The listing builds one solid part. Answer for the finished solid, in the listing's coordinates (mm). A direction names the side the tool comes from. Give positions to 0.01 mm unless a question says otherwise; leave off trailing zeros. Loops run counter-clockwise (first coordinate to the right, second up) from the corner with the lowest first, then second, coordinate; pieces in that order, holes last.
Item 1: The mould has two halves that part along X. Classify faces 1 (the face through (-6.43, 3.77, -7.44)), 2 (the face through (0, 2.8, 0)), 3 (the face through (4, 0, 0)): pulls with the +X half, pulls with the -X half, needs draft (parallel to the pull), parting line crosses it, or undercut.
Item 2: Each of these flat-tipped pins is pushed along its axis until it touches: pin 1 Ø0.5 at (y, z) = (0.5, 2) entering from -X; pin 2 Ø1 at (x, z) = (6, 1) entering from +Y; pin 3 Ø1.4 at (y, z) = (2, 1) entering from +X. Where does it stop, or does it pass through?
Item 3: Section B-B, the plane z = 0.5 is taken. Give the vertices of the cut face in (x, y), and give its area (3 significant figures).
Item 4: A tool of negligible diameter and unlimited length cuts with its end or side. For faces 4 (the face through (-6.43, 3.77, 7.44)), 5 (the face through (1.95, 2, 0)), 6 (the face through (2, 6, -1.5)), 7 (the face through (0, 3, -7.5)), 8 (the face through (2, 6, 1.5)), from which of +Z, -Z, +X, -X, +Y, -Y can it reach the whole face along a straight path? Write none if from no direction.
Item 5: Consider line 1 along Z through (x, y) = (1.25, 6.25); line 2 along Y through (x, z) = (1, -1.75); line 3 along X through (y, z) = (2, -5). Determine where each line is inside the solid, lowest interval first.
Item 6: Section A-A, the plane z = 2.75 is taken. Give the vertices of the cut face in (x, y).
from build123d import *

# Parameters (mm, degrees)
EXTRUDE_1_DEPTH      = 7.5
EXTRUDE_1_DEPTH_BACK = 7.5
EXTRUDE_2_DEPTH      = 1.5
EXTRUDE_2_DEPTH_BACK = 1.5
EXTRUDE_3_DEPTH      = 2
EXTRUDE_3_DEPTH_BACK = 2
CUT_EXTRUDE_1_DEPTH  = 16.207955299
FILLET_1_R           = 0.2
FILLET_2_R           = 0.1


with BuildPart() as part:
    # 草图1 → 凸台-拉伸1 (new, two sides: drawn at the far end of the back side and taken through both)
    with BuildSketch(Plane.XY.offset(-EXTRUDE_1_DEPTH_BACK)):
        with BuildLine():
            Line((-7.5, 0), (-1.5, 0))
            Line((-1.5, 0), (-1.5, 0.677124344))
            ThreePointArc((-1.5, 0.677124344), (-1.780042303, 1.088161527), (-1.95, 1.555590279))
            Line((-1.95, 1.555590279), (-1.95, 2.8))
            Line((-1.95, 2.8), (1.95, 2.8))
            Line((1.95, 2.8), (1.95, 1.555590279))
            ThreePointArc((1.95, 1.555590279), (1.780042303, 1.088161527), (1.5, 0.677124344))
            Line((1.5, 0.677124344), (1.5, 0))
            Line((1.5, 0), (7.5, 0))
            Line((7.5, 0), (8.53527618, 3.863703305))
            Line((8.53527618, 3.863703305), (-5.459914348, 7.613703305))
            Line((-5.459914348, 7.613703305), (-7.5, 0))
        make_face()
    extrude(amount=EXTRUDE_1_DEPTH + EXTRUDE_1_DEPTH_BACK)

    # 草图2 → 凸台-拉伸2 (add, two sides: drawn at the far end of the back side and taken through both)
    with BuildSketch(Plane.XY.offset(-EXTRUDE_2_DEPTH_BACK)):
        Polygon((0.088792177, 6.126931873), (2.986569656, 5.350474738), (3.245388701, 6.316400564), (0.347611222, 7.092857699), align=None)
    extrude(amount=EXTRUDE_2_DEPTH + EXTRUDE_2_DEPTH_BACK)

    # 草图3 → 凸台-拉伸3 (add, two sides: drawn at the far end of the back side and taken through both)
    with BuildSketch(Plane.XY.offset(-EXTRUDE_3_DEPTH_BACK)):
        with BuildLine():
            Line((2.184728529, 8.153517871), (4.06828389, 7.648820733))
            Line((4.06828389, 7.648820733), (3.823852668, 6.736590993))
            ThreePointArc((3.823852668, 6.736590993), (3.538706676, 6.329077778), (3.161822332, 6.004526629))
            Line((3.161822332, 6.004526629), (0.264044853, 6.780983765))
            ThreePointArc((0.264044853, 6.780983765), (0.099929011, 7.250495477), (0.056741946, 7.745985269))
            Line((0.056741946, 7.745985269), (0.301173168, 8.658215009))
            Line((0.301173168, 8.658215009), (2.184728529, 8.153517871))
        make_face()
    extrude(amount=EXTRUDE_3_DEPTH + EXTRUDE_3_DEPTH_BACK)

    # 草图4 → 切除-拉伸1 (cut, through all)
    with BuildSketch(Plane(origin=(-1.883555361, 0.504697138, 0), x_dir=(0, 0, 1), z_dir=(-0.9659258262890692, 0.2588190451025178, 0))):
        with BuildLine():
            Line((1.95, 8.441142838), (2, 8.441142838))
            Line((2, 8.441142838), (2, 6.618267183))
            Line((2, 6.618267183), (1.5, 6.618267183))
            ThreePointArc((1.5, 6.618267183), (1.780042303, 7.029304366), (1.95, 7.496733117))
            Line((1.95, 7.496733117), (1.95, 8.441142838))
        make_face()
        with BuildLine():
            Line((-1.95, 8.441142838), (-1.95, 7.496733117))
            ThreePointArc((-1.95, 7.496733117), (-1.780042303, 7.029304366), (-1.5, 6.618267183))
            Line((-1.5, 6.618267183), (-2, 6.618267183))
            Line((-2, 6.618267183), (-2, 8.441142838))
            Line((-2, 8.441142838), (-1.95, 8.441142838))
        make_face()
    extrude(amount=-CUT_EXTRUDE_1_DEPTH, mode=Mode.SUBTRACT)

    # 圆角1
    fillet_1_edges = [part.edges().sort_by_distance(p)[0] for p in [
        (-5.459914348, 7.613703305, 0),
        (8.53527618, 3.863703305, 0),
        (7.5, 0, 0),
        (1.5, 0, 0),
        (-1.5, 0, 0),
        (-7.5, 0, 0),
        (4.5, 0, -7.5),
        (-6.479957174, 3.806851653, 7.5),
        (-4.5, 0, 7.5),
        (8.01763809, 1.931851653, -7.5),
        (4.5, 0, 7.5),
        (8.01763809, 1.931851653, 7.5),
        (1.537680916, 5.738703305, 7.5),
        (1.537680916, 5.738703305, -7.5),
        (-6.479957174, 3.806851653, -7.5),
        (-4.5, 0, -7.5),
    ]]
    fillet(fillet_1_edges, radius=FILLET_1_R)

    # 圆角2
    fillet_2_edges = [part.edges().sort_by_distance(p)[0] for p in [
        (4.06828389, 7.648820733, 0),
        (0.301173168, 8.658215009, 0),
        (2.184728529, 8.153517871, -1.95),
        (2.184728529, 8.153517871, 1.95),
    ]]
    fillet(fillet_2_edges, radius=FILLET_2_R)


solid = part.part
Worked answers:
1. face 1: pulls with the -X half
1. face 2: undercut
1. face 3: needs draft
2. pin 1: stops at x = -7.43
2. pin 2: stops at y = 4.68
2. pin 3: stops at x = 8.22
3. outline: (-7.43, 0.25) arc R0.2 ccw to (-7.24, 0) - (-1.7, 0) arc R0.2 ccw to (-1.5, 0.2) - (-1.5, 0.68) arc R2 cw to (-1.95, 1.56) - (-1.95, 2.8) - (1.95, 2.8) - (1.95, 1.56) arc R2 cw to (1.5, 0.68) - (1.5, 0.2) arc R0.2 ccw to (1.7, 0) - (7.35, 0) arc R0.2 ccw to (7.54, 0.15) - (8.48, 3.67) arc R0.2 ccw to (8.34, 3.92) - (2.99, 5.35) - (3.16, 6) arc R2 ccw to (3.82, 6.74) - (4.04, 7.55) arc R0.1 ccw to (3.97, 7.67) - (0.4, 8.63) arc R0.1 ccw to (0.28, 8.56) - (0.06, 7.75) arc R2 ccw to (0.26, 6.78) - (0.09, 6.13) - (-5.27, 7.56) arc R0.2 ccw to (-5.51, 7.42) - close
3. area: 84.9 mm2
4. face 4: +Z, -X, +Y
4. face 5: +Z, -Z
4. face 6: -Z
4. face 7: -Z, +X, -X, +Y, -Y
4. face 8: +Z
5. line 1: z = -1.5 to 1.5
5. line 2: y = 2.8 to 5.88, 6.95 to 8.47
5. line 3: x = -6.96 to -1.95, 1.95 to 8.04
6. outline: (-7.43, 0.25) arc R0.2 ccw to (-7.24, 0) - (-1.7, 0) arc R0.2 ccw to (-1.5, 0.2) - (-1.5, 0.68) arc R2 cw to (-1.95, 1.56) - (-1.95, 2.8) - (1.95, 2.8) - (1.95, 1.56) arc R2 cw to (1.5, 0.68) - (1.5, 0.2) arc R0.2 ccw to (1.7, 0) - (7.35, 0) arc R0.2 ccw to (7.54, 0.15) - (8.48, 3.67) arc R0.2 ccw to (8.34, 3.92) - (-5.27, 7.56) arc R0.2 ccw to (-5.51, 7.42) - close
